from build123d import *

# Parameters (mm, degrees)
F0_W     = 26
F0_H     = 7
F0_R     = 1.45
F1_DEPTH = 6
F2_W     = 5
F2_H     = 25
F2_R     = 1.6
F3_DEPTH = 3
F4_SIZE  = 1
F6_DEPTH = 2


# Not quite as in the source:
# - a feature of the source that left no trace in its solid (it failed there, or was rolled back) is left out


with BuildPart() as f1:
    # F0 (on Top) → F1 (new body)
    with BuildSketch(Plane.XY):
        with Locations((-13, 3.5)):
            Rectangle(F0_W, F0_H)
        with Locations((-22.5, 4.5)):
            Circle(F0_R, mode=Mode.SUBTRACT)
        with Locations((-3.5, 4.5)):
            Circle(F0_R, mode=Mode.SUBTRACT)
    extrude(amount=F1_DEPTH)

    # F2 (on Top) → F3 (join)
    with BuildSketch(Plane.XY):
        with Locations((1.5, 3.5)):
            Rectangle(F2_W, F2_H)
        with Locations((-3.5, 3.5)):
            Rectangle(F2_W, F2_H)
        with Locations((-3.5, -5)):
            Circle(F2_R, mode=Mode.SUBTRACT)
        with Locations((-3.5, 12)):
            Circle(F2_R, mode=Mode.SUBTRACT)
        with Locations((-8.5, 3.5)):
            Rectangle(F2_W, F2_H)
    extrude(amount=-F3_DEPTH)

    # F4
    f4_edges = [f1.edges().sort_by_distance(p)[0] for p in [
        (4, 16, -1.5),
        (-11, 16, -1.5),
        (4, -9, -1.5),
        (-11, -9, -1.5),
    ]]
    chamfer(f4_edges, length=F4_SIZE)

    # F6 (cut): a face of the model
    f6_faces = [f1.faces().sort_by_distance(p)[0] for p in [
        (-18.2314818077, 3.4328704519, 0),
    ]]
    extrude(f6_faces, amount=-F6_DEPTH, mode=Mode.SUBTRACT)


solid = f1.part
CAD build for the part. Positions are in the model's coordinates, mm. A direction names the side the tool comes from. Round coordinates to 2 decimals unless told otherwise and drop trailing zeros. Write each loop counter-clockwise with the first axis right and the second up, starting at its lowest first coordinate (ties: lowest second). Pieces come first, ordered by that corner, then holes.
(1) Probe line 1 along Y through (x, z) = (-3.5, -1.15); line 2 along Z through (x, y) = (-4.5, -6.5); line 3 along Y through (x, z) = (-11.75, 5.75). List the from-to ranges inside material, lowest first.
(2) Drop flat-ended pins along their axis: P1, Ø3.5, axis at x = -15.5, y = 3.5, coming from the -Z side; P2, Ø2.5, axis at x = -3.5, y = -5, coming from the +Z side; P3, Ø5, axis at x = -3.5, y = 12, coming from the +Z side; P4, Ø1, axis at y = 11.5, z = -1, coming from the -X side. Give the stop position or say it passes through.
(3) Slice it at D-D, the plane z = 0.5. Write the cut outline in (x, y).
(4) Slice it at B-B, the plane x = -3.5. Write the cut outline in (y, z).
(5) 3-axis set-ups, long thin cutter, end or side, ignore diameter. For faces 1 (the face through (-4.65, 3.62, 2.96)), 2 (the face through (0, 3, 3)), 3 (the face through (-13, 7, 4)): which of +Z, -Z, +X, -X, +Y, -Y reach the whole face in a straight line?
(6) Mould opens along X. For faces 4 (the face through (4, 3, -1)), 5 (the face through (-4, 4, -3)), 6 (the face through (-4, 5, 0)) say: pulls with the +X half, pulls with the -X half, needs draft (parallel to the pull), parting line crosses it, or undercut.
(7) Slice it at C-C, the plane z = -2.5. Write the cut outline in (x, y).
(8) Slice it at A-A, the plane y = 4.5. Write the cut outline in (x, z), and give its area (3 significant figures).
From the geometry:
1. line 1: y = -9 to -6.6, -3.4 to 10.4, 13.6 to 16
1. line 2: z = -3 to 0
1. line 3: y = 0 to 7
2. P1: stops at z = 2
2. P2: passes through
2. P3: stops at z = 0
2. P4: stops at x = -11
3. outline: (-11, 0) - (0, 0) - (0, 7) - (-11, 7) - close; hole circle Ø2.9 at (-3.5, 4.5)
4. outline: (-9, -3) - (-6.6, -3) - (-6.6, 0) - (-9, 0) - close; (-3.4, -3) - (10.4, -3) - (10.4, 0) - (7, 0) - (7, 6) - (5.95, 6) - (5.95, 0) - (3.05, 0) - (3.05, 6) - (0, 6) - (0, 0) - (-3.4, 0) - close; (13.6, -3) - (16, -3) - (16, 0) - (13.6, 0) - close
5. face 1: +Z
5. face 2: +Z, +X, +Y, -Y
5. face 3: +Z, +X, -X, +Y
6. face 4: pulls with the +X half
6. face 5: needs draft
6. face 6: undercut
7. outline: (-11, -8) - (-10, -9) - (3, -9) - (4, -8) - (4, 15) - (3, 16) - (-10, 16) - (-11, 15) - close; hole circle Ø3.2 at (-3.5, -5); hole circle Ø3.2 at (-3.5, 12)
8. outline: (-26, 2) - (-23.95, 2) - (-23.95, 6) - (-26, 6) - close; (-21.05, 2) - (-11, 2) - (-11, -3) - (4, -3) - (4, 0) - (0, 0) - (0, 6) - (-2.05, 6) - (-2.05, 0) - (-4.95, 0) - (-4.95, 6) - (-21.05, 6) - close
8. area: 142 mm2
